Read the model definition and answer for the solid it produces. Units are mm, in the model's axes. A direction names the side the tool comes from. Give positions to 0.01 mm unless a question says otherwise; leave off trailing zeros. Order: outer loops, then holes, each group sorted by start corner. A loop starts at its lowest first (then second) coordinate and runs counter-clockwise, first axis right, second up.
```python
from build123d import *

# Parameters (mm, degrees)
BOSS_EXTRUDE1_DEPTH = 115
RIB1_REACH          = 191.225
SKETCH2_WALL_W      = 510.73669158
SKETCH2_WALL_H      = 10


with BuildPart() as part:
    # Sketch1 → Boss-Extrude1 (new body)
    with BuildSketch(Plane.XY):
        Polygon((0, 0), (0, 100), (150, 100), (150, 70), (50, 70), (50, 0), align=None)
    extrude(amount=BOSS_EXTRUDE1_DEPTH)

    # Sketch2 wall → Rib1 (add, up to next)
    with BuildSketch(Plane(origin=(78.259342081, 44.734908946, 57.5), x_dir=(0.80823649623, 0.588858018679, 0), z_dir=(-0.588858018679, 0.80823649623, 0)), mode=Mode.PRIVATE) as rib1_sk1:
        Rectangle(SKETCH2_WALL_W, SKETCH2_WALL_H)
    rib1_tool1 = extrude(rib1_sk1.sketch, amount=RIB1_REACH, mode=Mode.PRIVATE) - part.part
    add(rib1_tool1.solids().sort_by_distance((78.259342081, 44.734908946, 57.5))[0])


solid = part.part
```
1) Given pin 1 (2 mm diameter, centred on x = 45, y = 80.5, fed in from -Z); pin 2 (8 mm diameter, centred on x = 107, z = 18, fed in from -Y), each flat-ended and moving along its own axis, determine where each tip first touches the part or whether it passes through.
Final values:
pin 1: stops at z = 0
pin 2: stops at y = 70
2) The part is cut by section B-B on x = 59. Determine the outline of the cut face in (y, z).
Final values:
outline: (30.7, 52.5) - (70, 52.5) - (70, 0) - (100, 0) - (100, 115) - (70, 115) - (70, 62.5) - (30.7, 62.5) - close
3) The part is cut by section D-D on y = 9.5. Determine the outline of the cut face in (x, z), and give its area (3 significant figures).
Final values:
outline: (0, 0) - (50, 0) - (50, 115) - (0, 115) - close
area: 5,750 mm2
4) A tool of negligible diameter and unlimited length cuts with its end or side. For faces 1 (the face through (101, 70, 44)), 2 (the face through (73, 58, 62.5)), 3 (the face through (73, 58, 52.5)), from which of +Z, -Z, +X, -X, +Y, -Y can it reach the whole face along a straight path? Write none if from no direction.
Final values:
face 1: +X, -Y
face 2: +Z, +X, -Y
face 3: -Z, +X, -Y
5) The part is cut by section A-A on z = 58. Determine the outline of the cut face in (x, y).
Final values:
outline: (0, 0) - (50, 0) - (50, 24.15) - (112.94, 70) - (150, 70) - (150, 100) - (0, 100) - close
6) The part is cut by section C-C on y = 30. Determine the outline of the cut face in (x, z).
Final values:
outline: (0, 0) - (50, 0) - (50, 52.5) - (58.03, 52.5) - (58.03, 62.5) - (50, 62.5) - (50, 115) - (0, 115) - close
7) Consider L1, parallel to X at y = 47.5, z = 89.5; L2, parallel to Y at x = 103, z = 106; L3, parallel to Z at x = 67, y = 39.5. Determine where each line is inside the solid, lowest interval first.
Final values:
L1: x = 0 to 50
L2: y = 70 to 100
L3: z = 52.5 to 62.5
